Design review of the part built by this model. Coordinates are the model's own, in mm. Give positions to 0.01 mm unless a question says otherwise; leave off trailing zeros. Order: outer loops, then holes, each group sorted by start corner. A loop starts at its lowest first (then second) coordinate and runs counter-clockwise, first axis right, second up. Notation, with made-up numbers: (24.5, 40.5) -> (83.5, 40.5) arc R11 cw to (83.5, 56.5) -> close; hole circle Ø5 at (-26, 23.25). An arc over 180 degrees is marked (long way). One line per item, written item: value. Start each with the question number.
1) Consider section A-A (z = -13.5). State the section outline as (x, y) points (3 decimals).
2) Consider section C-C (y = 14.5). State the section outline as (x, z) points (3 decimals).
3) For pin 1 (10 mm diameter, centred on y = 25.5, z = -3.5, fed in from +X) (3 decimals); pin 2 (0.6 mm diameter, centred on x = 1, z = -29, fed in from +Y); pin 3 (1.6 mm diameter, centred on x = 2, z = -5, fed in from +Y); pin 4 (1 mm diameter, centred on x = 2, y = 14.5, fed in from -Z), all flat-tipped, find the tip position at first contact; note any pin that passes through.
4) Wall thickness on line 1 along Y through (x, z) = (1.25, -18) (3 decimals); line 2 along Y through (x, z) = (3, -15.5) (3 decimals); line 3 along Z through (x, y) = (1.25, 3): over which ranges is each line inside the solid? List them lowest first. Write a range as from..to.
5) Consider section D-D (z = -26.5). State the section outline as (x, y) points (3 decimals).
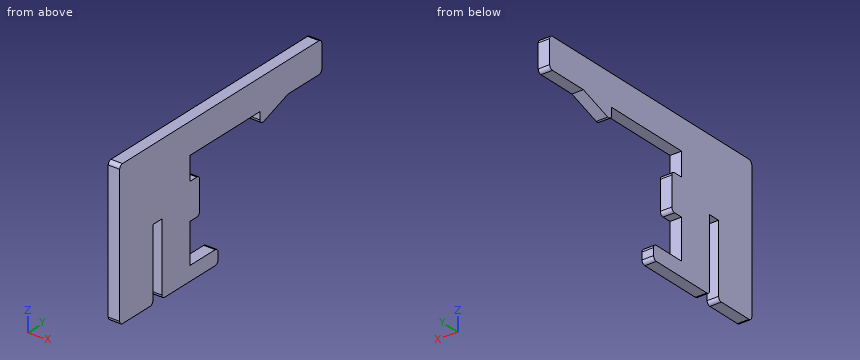
from build123d import *

# Parameters (mm, degrees)
BOSS_EXTRUDE1_DEPTH = 3.175
FILLET1_R           = 1


with BuildPart() as part:
    # Sketch1 → Boss-Extrude1 (new body)
    with BuildSketch(Plane(origin=(0, 0, 0), x_dir=(0, 0, -1), z_dir=(1, 0, 0))):
        Polygon((0, 47), (-8.5, 47), (-8.5, -10), (31.5, -10), (31.5, 10), (27.5, 10), (27.5, 0), (16.5, 0), (16.5, 3.5), (6.5, 3.5), (6.5, 0), (0, 0), (0, 25), (3.5, 25), (0, 35), align=None)
        Polygon((11.5, -10), (-8.5, -10), (-8.5, -25), (31.5, -25), (31.5, -13.175), (11.5, -13.175), align=None)
    extrude(amount=BOSS_EXTRUDE1_DEPTH)

    # Fillet1
    fillet1_edges = [part.edges().sort_by_distance(p)[0] for p in [
        (1.5875, 47, 0),
        (1.5875, 25, -3.5),
        (1.5875, 3.5, -6.5),
        (1.5875, 3.5, -16.5),
        (1.5875, 10, -27.5),
        (1.5875, 10, -31.5),
        (1.5875, -10, -31.5),
        (1.5875, -13.175, -31.5),
        (1.5875, -25, -31.5),
        (1.5875, -25, 8.5),
        (1.5875, 47, 8.5),
    ]]
    fillet(fillet1_edges, radius=FILLET1_R)


solid = part.part
Checked values:
1. outline: (0, -25) -> (3.175, -25) -> (3.175, -13.175) -> (0, -13.175) -> close; (0, -10) -> (3.175, -10) -> (3.175, 3.5) -> (0, 3.5) -> close
2. outline: (0, 0) -> (3.175, 0) -> (3.175, 8.5) -> (0, 8.5) -> close
3. pin 1: stops at x = 3.175
3. pin 2: stops at y = 10
3. pin 3: stops at y = 0
3. pin 4: stops at z = 0
4. line 1: y = -25..-13.175, -10..0
4. line 2: y = -25..-13.175, -10..3.5
4. line 3: z = -31.5..-27.5, -16.37..-6.63, 0..8.5
5. outline: (0, -25) -> (3.175, -25) -> (3.175, -13.175) -> (0, -13.175) -> close; (0, -10) -> (3.175, -10) -> (3.175, 0) -> (0, 0) -> close
